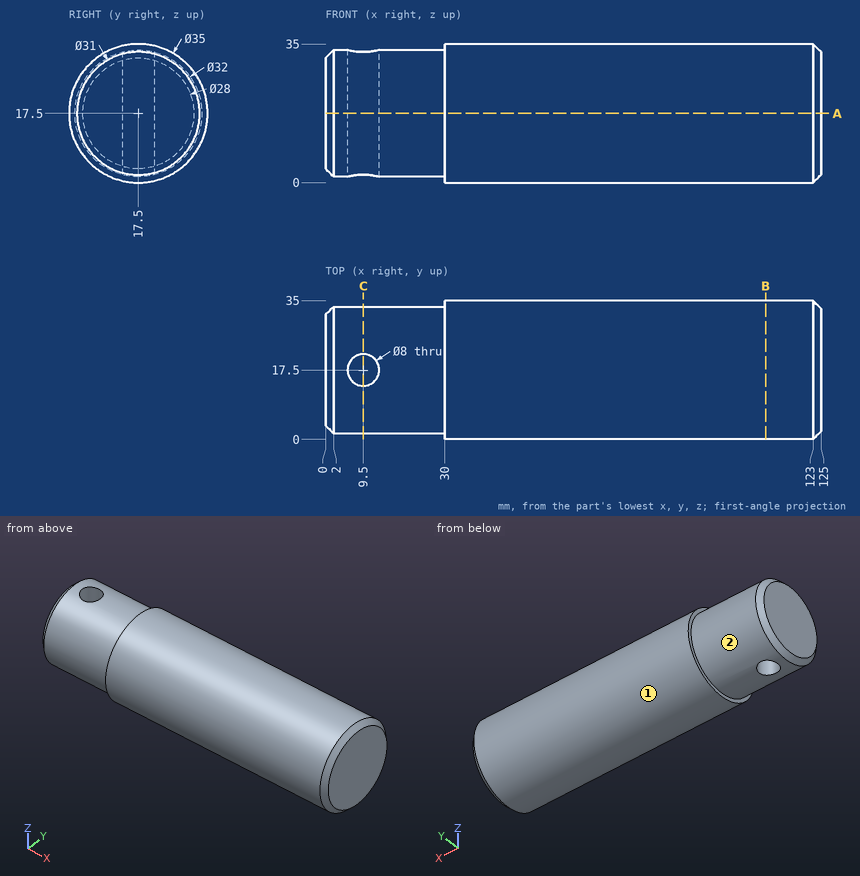
Can you work these out from the drawing? Everything is in mm from the part's minimum corner. A direction names the side the tool comes from. Round coordinates to 2 decimals unless told otherwise and drop trailing zeros. Loops run counter-clockwise (first coordinate to the right, second up) from the corner with the lowest first, then second, coordinate; pieces in that order, holes last. Notation, with made-up numbers: M -6.5,67.25 L 3.5,67.25 A16 cw 3.5,79.25 Z; hole C -4,-19 d11. An arc over 180 degrees is marked long. Write item = value, one per line.
1. Which directions (+Z, -Z, +X, -X, +Y, -Y) give clear straight access to the entire face, cutting with the end or side of a thin tool? Please do the marked faces 1 and 2.
Results below:
face_1 = +X, -X
face_2 = -X
2. I want a section at A-A, the plane z = 17.5. Write out the boundary of the cut face in (x, y).
Results below:
outline = M 0,3.5 L 2,1.5 L 30,1.5 L 30,0 L 123,0 L 125,2 L 125,33 L 123,35 L 30,35 L 30,33.5 L 2,33.5 L 0,31.5 Z; hole C 9.5,17.5 d8
3. Will these pins go through, and if not, where does the flat tip stop? P1, Ø2, axis at y = 8.5, z = 20.5, coming from the -X side; P2, Ø4, axis at x = 32, y = 21, coming from the +Z side; P3, Ø6, axis at x = 18.5, y = 6.5, coming from the +Z side; P4, Ø6, axis at x = 31, z = 21, coming from the -Y side.
Results below:
P1 = 0
P2 = 34.94
P3 = 31.36
P4 = 0.01
4. I want a section at C-C, the plane x = 9.5. Write out the boundary of the cut face in (y, z), and give its area (3 significant figures).
Results below:
outline = M 13.5,2.01 L 13.5,32.99 A16 ccw Z; M 21.5,2.01 A16 ccw 21.5,32.99 Z
area = 551 mm²
5. I want a section at B-B, the plane x = 111. Write out the boundary of the cut face in (y, z).
Results below:
outline = C 17.5,17.5 d35
6. I need wall thicknesses on probe 1 along Y at (x, z) = (9.5, 21.5); probe 2 along X at (y, z) = (17.5, 14.5); probe 3 along Y at (x, z) = (9.5, 22). Which ranges of each line are inside material? Lowest first, please.
Results below:
probe_1 = 2.01 to 13.5, 21.5 to 32.99
probe_2 = 0 to 5.5, 13.5 to 125
probe_3 = 2.15 to 13.5, 21.5 to 32.85
